Input: part model. Units: mm. Frame: model coordinates. Face numbers are marked on the shaded views. A direction names the side the tool comes from. Coordinates: 2 decimals unless noted, no trailing zeros. Loops run counter-clockwise (first coordinate to the right, second up) from the corner with the lowest first, then second, coordinate; pieces in that order, holes last. Notation, with made-up numbers: (-0.75, -27.5) - (52.25, -27.5) arc R21 ccw to (52.25, -12.5) - close; hole circle Ø8 at (60, 63.25). An arc over 180 degrees is marked (long way). Use one line per item in the form item = value.
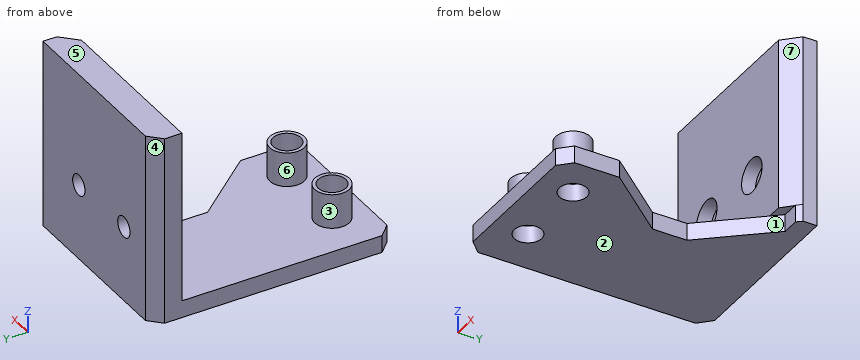
from build123d import *

# Parameters (mm, degrees)
BOSS_EXTRUDE1_DEPTH     = 5
BOSS_EXTRUDE2_DEPTH     = 50
CUT_EXTRUDE1_DEPTH      = 99.333615819
CUT_EXTRUDE1_DEPTH_BACK = 99.333615819
SKETCH3_R               = 3
SKETCH4_R               = 5
SKETCH4_R_2             = 4
BOSS_EXTRUDE3_DEPTH     = 10
SKETCH3_3_R             = 5
SKETCH3_3_R_2           = 3
CUT_EXTRUDE2_DEPTH      = 4
ESQUISSE1_R             = 4
ENL_V_MAT_EXTRU_1_DEPTH = 99.916631564


with BuildPart() as part:
    # Sketch1 → Boss-Extrude1 (new body)
    with BuildSketch(Plane.XY):
        Polygon((53.5, -0.5), (53.5, 3.5), (3.5, 3.5), (0, 0), (0, -63), (3.5, -66.5), (43.741350553, -66.5), (47.241350553, -63), (47.241350553, -50), (31.298457561, -31), (31.298457561, -21), (47.241350553, -2), (52.241350553, -2), align=None)
    extrude(amount=BOSS_EXTRUDE1_DEPTH)

    # Sketch2 → Boss-Extrude2 (add)
    with BuildSketch(Plane.XY.offset(5)):
        Polygon((0, -5), (0, 0), (3.5, 3.5), (53.5, 3.5), (53.5, -0.5), (49, -5), align=None)
    extrude(amount=BOSS_EXTRUDE2_DEPTH)

    # Sketch3 → Cut-Extrude1 (cut, two sides: drawn at the far end of the back side and taken through both)
    with BuildSketch(Plane.XZ.offset(5).offset(-CUT_EXTRUDE1_DEPTH_BACK)):
        with Locations((36, 22)):
            Circle(SKETCH3_R)
        with Locations((14, 22)):
            Circle(SKETCH3_R)
    extrude(amount=CUT_EXTRUDE1_DEPTH + CUT_EXTRUDE1_DEPTH_BACK, mode=Mode.SUBTRACT)

    # Sketch4 → Boss-Extrude3 (add)
    # profile 1 of 2: a face of its own
    with BuildSketch(Plane.XY.offset(5)):
        with Locations((13.5, -56.5)):
            Circle(SKETCH4_R)
        with Locations((13.5, -56.5)):
            Circle(SKETCH4_R_2, mode=Mode.SUBTRACT)
    # profile 2 of 2: a face of its own
    with BuildSketch(Plane.XY.offset(5)):
        with Locations((35.5, -56.5)):
            Circle(SKETCH4_R)
        with Locations((35.5, -56.5)):
            Circle(SKETCH4_R_2, mode=Mode.SUBTRACT)
    extrude(amount=BOSS_EXTRUDE3_DEPTH)

    # Sketch3_3 → Cut-Extrude2 (cut)
    # profile 1 of 2: a face of its own
    with BuildSketch(Plane.XZ.offset(5)):
        with Locations((36, 22)):
            Circle(SKETCH3_3_R)
        with Locations((36, 22)):
            Circle(SKETCH3_3_R_2, mode=Mode.SUBTRACT)
    # profile 2 of 2: a face of its own
    with BuildSketch(Plane.XZ.offset(5)):
        with Locations((14, 22)):
            Circle(SKETCH3_3_R)
        with Locations((14, 22)):
            Circle(SKETCH3_3_R_2, mode=Mode.SUBTRACT)
    extrude(amount=-CUT_EXTRUDE2_DEPTH, mode=Mode.SUBTRACT)

    # Esquisse1 → Enl_v. mat.-Extru.1 (cut, through all)
    with BuildSketch(Plane.XY.offset(5)):
        with Locations((35.5, -56.5)):
            Circle(ESQUISSE1_R)
        with Locations((13.5, -56.5)):
            Circle(ESQUISSE1_R)
    extrude(amount=-ENL_V_MAT_EXTRU_1_DEPTH, mode=Mode.SUBTRACT)


solid = part.part
Q1. Set-up query: the marked faces 5, 6 and 7. Return all of +Z, -Z, +X, -X, +Y, -Y with unobstructed straight access to the full face (end or side cutting, diameter ignored); none if empty.
Check values:
face_5 = +Z, +X, -X, +Y, -Y
face_6 = +Z
face_7 = +Z, +X, -Y
Q2. Pull-direction query (Y, two-part tool) for the marked faces 1, 2, 3 and 4; classes: pulls with the +Y half, pulls with the -Y half, needs draft (parallel to the pull), parting line crosses it, or undercut.
Check values:
face_1 = undercut
face_2 = needs draft
face_3 = undercut
face_4 = pulls with the +Y half
Q3. First-contact query: P1, Ø5.5, axis at y = -28, z = 1.5, coming from the +X side; P2, Ø3, axis at x = 43.5, z = 7, coming from the -Y side; P3, Ø1.5, axis at x = 5.5, y = -58.5, coming from the +Z side. Flat tips, straight axial feed; report the tip coordinate or a pass-through.
Check values:
P1 = 31.3
P2 = -5
P3 = 5
Q4. Ray query, line 1 along Y through (x, z) = (13.5, 9.75); line 2 along Y through (x, z) = (13.5, 2.9); line 3 along Z through (x, y) = (14, -3.4). Return the intervals inside material, ascending. Write a range as [from, to].
Check values:
line_1 = [-61.5, -60.5], [-52.5, -51.5], [-5, 3.5]
line_2 = [-66.5, -60.5], [-52.5, 3.5]
line_3 = [0, 17], [27, 55]
Q5. Cut plane D-D, the plane x = 13.5. Return loops of the section in (y, z), then the cut area to 3 significant figures.
Check values:
outline = (-66.5, 0) - (-60.5, 0) - (-60.5, 15) - (-61.5, 15) - (-61.5, 5) - (-66.5, 5) - close; (-52.5, 0) - (3.5, 0) - (3.5, 19.04) - (-1, 19.04) - (-1, 17.03) - (-5, 17.03) - (-5, 5) - (-51.5, 5) - (-51.5, 15) - (-52.5, 15) - close; (-5, 26.97) - (-1, 26.97) - (-1, 24.96) - (3.5, 24.96) - (3.5, 55) - (-5, 55) - close
area = 689 mm²
Q6. Cut plane B-B, the plane x = 35.5. Return loops of the section in (y, z).
Check values:
outline = (-66.5, 0) - (-60.5, 0) - (-60.5, 15) - (-61.5, 15) - (-61.5, 5) - (-66.5, 5) - close; (-52.5, 0) - (-36.01, 0) - (-36.01, 5) - (-51.5, 5) - (-51.5, 15) - (-52.5, 15) - close; (-15.99, 0) - (3.5, 0) - (3.5, 19.04) - (-1, 19.04) - (-1, 17.03) - (-5, 17.03) - (-5, 5) - (-15.99, 5) - close; (-5, 26.97) - (-1, 26.97) - (-1, 24.96) - (3.5, 24.96) - (3.5, 55) - (-5, 55) - close
Q7. Cut plane A-A, the plane y = -56.5. Return loops of the section in (x, z).
Check values:
outline = (0, 0) - (9.5, 0) - (9.5, 15) - (8.5, 15) - (8.5, 5) - (0, 5) - close; (17.5, 0) - (31.5, 0) - (31.5, 15) - (30.5, 15) - (30.5, 5) - (18.5, 5) - (18.5, 15) - (17.5, 15) - close; (39.5, 0) - (47.24, 0) - (47.24, 5) - (40.5, 5) - (40.5, 15) - (39.5, 15) - close
Q8. Cut plane C-C, the plane z = 22. Return loops of the section in (x, y).
Check values:
outline = (0, -5) - (9, -5) - (9, -1) - (11, -1) - (11, 3.5) - (3.5, 3.5) - (0, 0) - close; (17, -1) - (19, -1) - (19, -5) - (31, -5) - (31, -1) - (33, -1) - (33, 3.5) - (17, 3.5) - close; (39, -1) - (41, -1) - (41, -5) - (49, -5) - (53.5, -0.5) - (53.5, 3.5) - (39, 3.5) - close
